```python
from build123d import *

# Parameters (mm, degrees)
F0_W     = 356
F0_H     = 98.5
F3_DEPTH = 10
F4_D     = 12
F5_D     = 10.5
F6_D     = 5.5


with BuildPart() as f3:
    # F0 (on Top) → F3 (new body)
    with BuildSketch(Plane.XY):
        with Locations((178, -49.25)):
            Rectangle(F0_W, F0_H)
    extrude(amount=F3_DEPTH)

    # F4 (through all)
    with Locations(Plane(origin=(0, 0, 0), x_dir=(1, 0, 0), z_dir=(0, 0, -1))):
        with Locations((75.5, 22.5), (75.5, 67.5), (280.5, 67.5), (280.5, 22.5)):
            Hole(F4_D / 2)

    # F5 (through all)
    with Locations(Plane(origin=(0, 0, 0), x_dir=(1, 0, 0), z_dir=(0, 0, -1))):
        with Locations((13, 11.9172791019), (43, 11.9172791019), (13, 71.9172791019), (43, 71.9172791019), (313, 11.9172791019), (343, 11.9172791019), (343, 71.9172791019), (313, 71.9172791019)):
            Hole(F5_D / 2)

    # F6 (through all)
    with Locations(Plane(origin=(0, 0, 0), x_dir=(1, 0, 0), z_dir=(0, 0, -1))):
        with Locations((158, 8), (198, 8), (158, 32), (198, 32)):
            Hole(F6_D / 2)


solid = f3.part
```
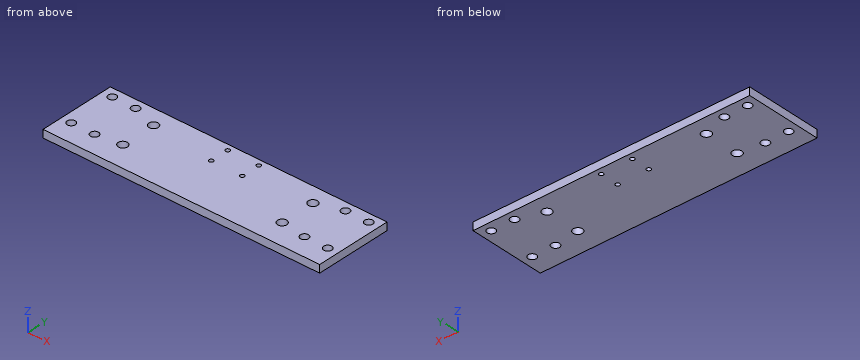
The listing builds one solid part. Answer for the finished solid, in the listing's coordinates (mm). Coordinates: 2 decimals unless noted, no trailing zeros. Loops run counter-clockwise (first coordinate to the right, second up) from the corner with the lowest first, then second, coordinate; pieces in that order, holes last. Notation, with made-up numbers: (9, -5) -> (30, -5) arc R12 ccw to (30, 11) -> close; hole circle Ø5 at (89.5, -38.5). An arc over 180 degrees is marked (long way). Use one line per item in the form item = value. Start each with the question number.
Item 1: The part is cut by section B-B on z = 4.75. Count the separate pieces of the cut face and the enclosed holes in it, then the cut area to 3 significant figures.
Item 2: The part is cut by section A-A on x = 280.5. Determine the outline of the cut face in (y, z), then the cut area to 3 significant figures.
Item 3: Consider L1, parallel to Y at x = 13, z = 3.5; L2, parallel to X at y = -32, z = 2; L3, parallel to Y at x = 198, z = 3.5. Determine where each line is inside the solid, lowest interval first. Write a range as [from, to].
Item 4: The part is cut by section C-C on x = 73. Determine the outline of the cut face in (y, z), then the cut area to 3 significant figures.
Answer key:
q1.separate_pieces = 1
q1.enclosed_holes = 16
q1.area = 33,800 mm2
q2.outline = (-98.5, 0) -> (-73.5, 0) -> (-73.5, 10) -> (-98.5, 10) -> close; (-61.5, 0) -> (-28.5, 0) -> (-28.5, 10) -> (-61.5, 10) -> close; (-16.5, 0) -> (0, 0) -> (0, 10) -> (-16.5, 10) -> close
q2.area = 745 mm2
q3.L1 = [-98.5, -77.17], [-66.67, -17.17], [-6.67, 0]
q3.L2 = [0, 155.25], [160.75, 195.25], [200.75, 356]
q3.L3 = [-98.5, -34.75], [-29.25, -10.75], [-5.25, 0]
q4.outline = (-98.5, 0) -> (-72.95, 0) -> (-72.95, 10) -> (-98.5, 10) -> close; (-62.05, 0) -> (-27.95, 0) -> (-27.95, 10) -> (-62.05, 10) -> close; (-17.05, 0) -> (0, 0) -> (0, 10) -> (-17.05, 10) -> close
q4.area = 767 mm2
